Work out the finished part from the listing and answer in its coordinate system (mm). A direction names the side the tool comes from. Give positions to 0.01 mm unless a question says otherwise; leave off trailing zeros. Loops run counter-clockwise (first coordinate to the right, second up) from the corner with the lowest first, then second, coordinate; pieces in that order, holes last. Notation, with made-up numbers: (66.5, 58.5) - (85.5, 58.5) arc R18 ccw to (85.5, 79.5) - close; hole circle Ø7 at (59, 9.25). An arc over 180 degrees is marked (long way). Use CSV: the item, a comma, the result in double quotes.
Autodesk Inventor part; units mm, degrees
ref_plane "YZ Plane" through (0, 0, 0) normal (1, 0, 0) x (0, 1, 0)
ref_plane "XZ Plane" through (0, 0, 0) normal (0, 1, 0) x (-1, 0, 0)
ref_plane "XY Plane" through (0, 0, 0) normal (0, 0, 1) x (1, 0, 0)
sketch "Эскиз1" plane through (0, 0, 0) normal (1, 0, 0) x (0, 1, 0)
  line L0 (-14, 0) -> (14, 0)
  line L1 (0, -56) -> (0, 56)
  line L2 (10, 40) -> (-10, 40)
  line L3 (-10, 40) -> (-10, -40)
  line L4 (-10, -40) -> (10, -40)
  line L5 (10, -40) -> (10, 40)
  point P0 (0, 0)
  dimension "d0" = 20
  dimension "d1" = 10
  dimension "d2" = 80
  dimension "d3" = 40
extrude "Выдавливание1" add sketch "Эскиз1" against normal blind 70
sketch "Эскиз2" plane through (0, 0, 0) normal (1, 0, 0) x (0, 1, 0)
  line L0 (0, 56) -> (0, -56)
  line L1 (0, -56) -> (0, 56)
  line L2 (-14, 0) -> (14, 0)
  circle A0 centre (0, 25) radius 5
  circle A1 centre (0, -25) radius 5
  line L3 (10, 40) -> (-10, 40)
  line L4 (-10, -40) -> (10, -40)
  point P0 (0, 0)
  dimension "d6" = 10
  dimension "d7" = 10
  dimension "d10" = 15
  dimension "d12" = 15
hole "Отверстие1" at (0, 0, 25) at (0, 0, -25) direction (-1, 0, 0) diameter 10.5 end through all counterbore diameter 18 counterbore depth 13.5
fillet "Сопряжение1" radius 5 2 edges at (0, 0, 40) (0, 0, -40)
chamfer "Фаска1" distance 1 angle 45 10 edges at (-37.5, 10, 40) (-1.4645, 10, 38.5355) (0, 10, 0) (-1.4645, 10, -38.5355) (-37.5, 10, -40) (-37.5, -10, 40) (-1.4645, -10, 38.5355) (0, -10, 0) (-1.4645, -10, -38.5355) (-37.5, -10, -40)
chamfer "Фаска2" distance 1 angle 45 4 edges at (-70, 10, 0) (-70, 0, 40) (-70, -10, 0) (-70, 0, -40)
sketch "Эскиз3" plane through (-70, 0, 0) normal (-1, 0, 0) x (0, 0, 1)
  line L0 (-56, 0) -> (56, 0)
  line L1 (0, 14) -> (0, -14)
  line L2 (-56, 0) -> (56, 0)
  circle A0 centre (-14, 0) radius 3
  circle A1 centre (14, 0) radius 3
  circle A2 centre (-25, 0) radius 5.25
  circle A3 centre (25, 0) radius 5.25
  point P0 (0, 0)
  dimension "d28" = 6
  dimension "d29" = 11
  dimension "d30" = 28
hole "Отверстие2" at (-70, 0, -14) at (-70, 0, 14) direction (1, 0, 0) diameter 6 depth 10 tip angle 118 countersink diameter 8 countersink angle 45
chamfer "Фаска3" distance 0.4 angle 45 2 edges at (-70, 0, -19.75) (-70, 0, 30.25)
sketch "Эскиз4" plane through (0, 0, 0) normal (0, 1, 0) x (-1, 0, 0)
  line L0 (69.6, 19.75) -> (13.5, 19.75)
  line L1 (69.6, -19.75) -> (13.5, -19.75)
  line L2 (70, -39) -> (70, 39)
  arc A0 (21, 7.5) -> (9, 7.5) centre (15, 7.5) ccw
  arc A1 (9, -7.5) -> (21, -7.5) centre (15, -7.5) ccw
  line L3 (15, 7.5) -> (15, -7.5) construction
  line L4 (-14, 0) -> (84, 0)
  line L5 (0, -56) -> (0, 56)
  line L6 (0, 25) -> (0, 25)
  line L7 (0, 25) -> (0, 25)
  line L8 (13.5, 34) -> (13.5, 16)
  line L9 (21, 7.5) -> (21, -7.5)
  line L10 (9, 7.5) -> (9, -7.5)
  point P0 (0, 0)
  dimension "d41" = 12
  dimension "d42" = 15
  dimension "d43" = 7.5
  dimension "d44" = 55
extrude "Выдавливание2" cut sketch "Эскиз4" along normal through all both and the other way through all
chamfer "Фаска4" distance 0.2 angle 45 8 edges at (-15, -10, 13.5) (-9, -10, 0) (-15, -10, -13.5) (-21, -10, 0) (-21, 10, 0) (-15, 10, -13.5) (-9, 10, 0) (-15, 10, 13.5)
properties part number "ОПОРА_01"
Item 1: The mould has two halves that part along Y. Classify faces 4 (the flat face through (-13.5, 4, -29)), 5 (the conical face through (-2.003, 9.715, -38.063)), 6 (the conical face through (-1.937, -9.715, -37.997)): pulls with the +Y half, pulls with the -Y half, needs draft (parallel to the pull), parting line crosses it, or undercut.
Determined:
face 4,"undercut"
face 5,"pulls with the +Y half"
face 6,"pulls with the -Y half"
Item 2: Given P1, Ø3.5, axis at y = 0, z = -14, coming from the +X side; P2, Ø5.5, axis at y = -3, z = -21.5, coming from the +X side, each flat-ended and moving along its own axis, determine where each tip first touches the part or whether it passes through.
Determined:
P1,"stops at x = 0"
P2,"stops at x = -13.5"
Item 3: A cutting plane is placed at A-A on x = -15. Determine the outline of the cut face in (y, z), and give its area (3 significant figures).
Determined:
outline,"(-10, -39) - (-9, -40) - (9, -40) - (10, -39) - (10, -13.7) - (9.8, -13.5) - (-9.8, -13.5) - (-10, -13.7) - close; (-10, 13.7) - (-9.8, 13.5) - (9.8, 13.5) - (10, 13.7) - (10, 39) - (9, 40) - (-9, 40) - (-10, 39) - close; hole circle Ø10.5 at (0, -25); hole circle Ø10.5 at (0, 25)"
area,"885 mm²"
Item 4: A cutting plane is placed at D-D on y = 7.5. Determine the outline of the cut face in (x, z).
Determined:
outline,"(-70, -39) - (-69, -40) - (-5, -40) arc R5 ccw to (0, -35) - (0, -29.97) - (-13.5, -29.97) - (-13.5, -20.03) - (0, -20.03) - (0, 20.03) - (-13.5, 20.03) - (-13.5, 29.97) - (0, 29.97) - (0, 35) arc R5 ccw to (-5, 40) - (-69, 40) - (-70, 39) - close; hole (-21, -7.5) arc R6 ccw to (-9, -7.5) - (-9, 7.5) arc R6 ccw to (-21, 7.5) - close"
Item 5: For faces 1 (the cylindrical face through (-64, 0, 11)), 2 (the flat face through (-35, -10, 1)), 3 (the flat face through (-21, 0, 0)), determine the directions among +Z, -Z, +X, -X, +Y, -Y from which every point of the face is accessible in a straight line to the end or side of a thin tool.
Determined:
face 1,"-X"
face 2,"+Z, -Z, +X, -X, -Y"
face 3,"+Y, -Y"
Item 6: A cutting plane is placed at C-C on x = -30. Determine the outline of the cut face in (y, z), and give its area (3 significant figures).
Determined:
outline,"(-10, -39) - (-9, -40) - (9, -40) - (10, -39) - (10, 39) - (9, 40) - (-9, 40) - (-10, 39) - close; hole circle Ø10.5 at (0, -25); hole circle Ø10.5 at (0, 25)"
area,"1,420 mm²"
Item 7: Find the intervals of material crossed by line 1 (Z direction, x = -50, y = 0); line 2 (Z direction, x = -64.25, y = 0); line 3 (Y direction, x = -7, z = 25), in increasing order.
Determined:
line 1,"z = -40 to -30.25, -19.75 to 19.75, 30.25 to 40"
line 2,"z = -40 to -30.25, -19.75 to -17, -11 to 11, 17 to 19.75, 30.25 to 40"
line 3,"y = -10 to -9, 9 to 10"
